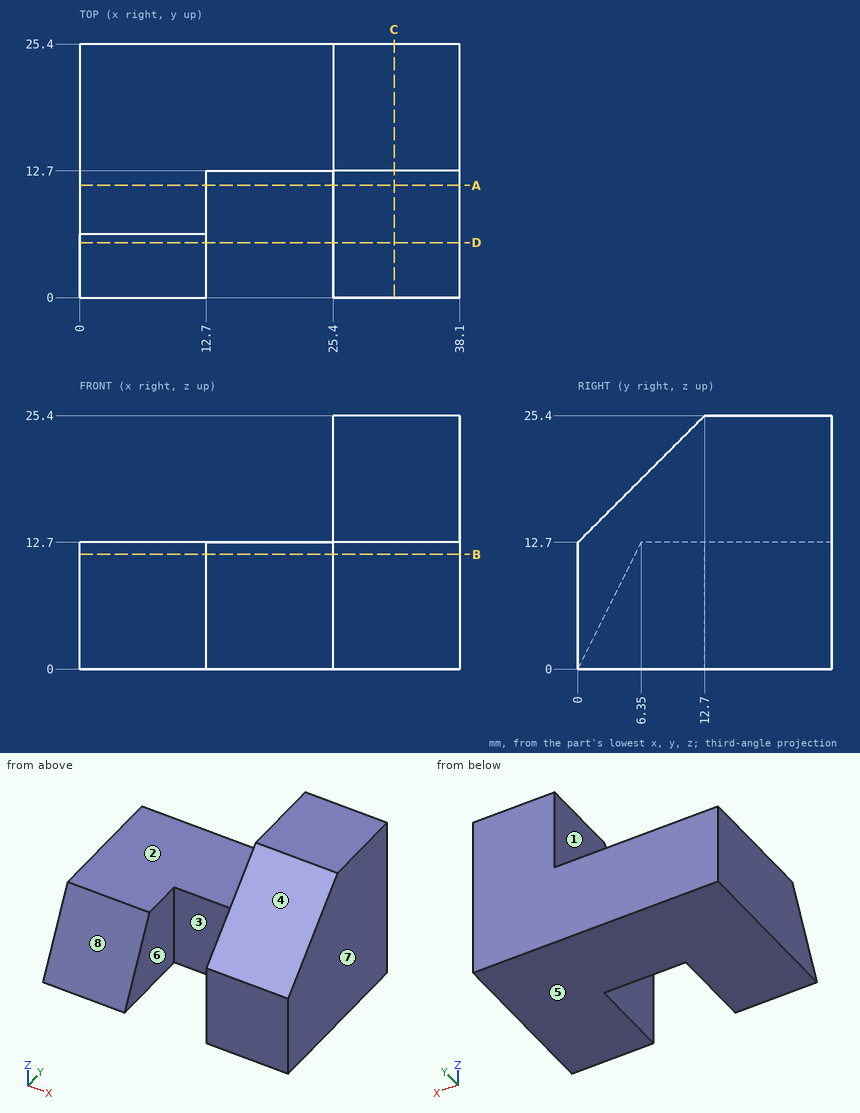
Job drawing, mm, ordinate dimensions from the low corner. One solid piece. A direction names the side the tool comes from. Coordinates: 2 decimals unless noted, no trailing zeros. Order: outer loops, then holes, each group sorted by start corner. A loop starts at its lowest first (then second) coordinate and runs counter-clockwise, first axis right, second up. Notation, with made-up numbers: M -36.5,86.5 L -25.5,86.5 A4 cw -25.5,90.5 Z; hole C 3.25,29 d6. An arc over 180 degrees is marked long. Answer as CSV lines item,"result".
(1) Wall check: line 1 along X through (y, z) = (7.75, 3); line 2 along X through (y, z) = (1.5, 12.75); line 3 along Z through (x, y) = (19, 14.5). Give the ranges that are in metal, low to high.
Geometry says:
line 1,"x = 0 to 12.7, 25.4 to 38.1"
line 2,"x = 25.4 to 38.1"
line 3,"z = 0 to 12.7"
(2) Band-saw the part on D-D, the plane y = 5.5. List the corners of the cut face in (x, z).
Geometry says:
outline,"M 0,0 L 12.7,0 L 12.7,11 L 0,11 Z; M 25.4,0 L 38.1,0 L 38.1,18.2 L 25.4,18.2 Z"
(3) Band-saw the part on A-A, the plane y = 11.25. List the corners of the cut face in (x, z).
Geometry says:
outline,"M 0,0 L 12.7,0 L 12.7,12.7 L 0,12.7 Z; M 25.4,0 L 38.1,0 L 38.1,23.95 L 25.4,23.95 Z"
(4) Pull direction X, two halves, no side cores. Call the marked faces 6, 7 and 8: +X half, -X half, draft (parallel to the pull), parting line (faces both ways), or undercut.
Geometry says:
face 6,"undercut"
face 7,"+X half"
face 8,"draft"
(5) Band-saw the part on B-B, the plane z = 11.5. List the corners of the cut face in (x, y).
Geometry says:
outline,"M 0,5.75 L 12.7,5.75 L 12.7,12.7 L 25.4,12.7 L 25.4,0 L 38.1,0 L 38.1,25.4 L 0,25.4 Z"
(6) Band-saw the part on C-C, the plane x = 31.5. List the corners of the cut face in (y, z), then the cut area to 3 significant figures.
Geometry says:
outline,"M 0,0 L 25.4,0 L 25.4,25.4 L 12.7,25.4 L 0,12.7 Z"
area,"565 mm2"
(7) 3-axis set-ups, long thin cutter, end or side, ignore diameter. For the marked faces 1, 2, 3, 4 and 5: which of +Z, -Z, +X, -X, +Y, -Y reach the whole face in a straight line?
Geometry says:
face 1,"+Z, -Y"
face 2,"+Z, -X, +Y, -Y"
face 3,"+Z, -Z, -Y"
face 4,"+Z, +X, -X, -Y"
face 5,"-Z, +X, -X, +Y, -Y"
(8) Flat gauge pins, fed straight in: pin 1 (5 mm diameter, centred on x = 16.5, y = 11, fed in from +Z); pin 2 (2 mm diameter, centred on x = 21, z = 10, fed in from -Y); pin 3 (1 mm diameter, centred on x = 7.5, z = 3.5, fed in from -Y). Where does each tip first touch, or does it go through?
Geometry says:
pin 1,"stops at z = 12.7"
pin 2,"stops at y = 12.7"
pin 3,"stops at y = 1.5"
